Autodesk Inventor part; units mm, degrees
ref_plane "YZ Plane" through (0, 0, 0) normal (1, 0, 0) x (0, 1, 0)
ref_plane "XZ Plane" through (0, 0, 0) normal (0, 1, 0) x (-1, 0, 0)
ref_plane "XY Plane" through (0, 0, 0) normal (0, 0, 1) x (1, 0, 0)
sketch "Sketch1" plane through (0, 0, 0) normal (0, 1, 0) x (-1, 0, 0)
  circle A0 centre (0, 0) radius 8
  dimension "d0" = 16
extrude "Extrusion1" add sketch "Sketch1" along normal blind 7.1
sketch "Sketch2" plane through (0, 7.1, 0) normal (0, 1, 0) x (1, 0, 0)
  circle A0 centre (0, 0) radius 6
  dimension "d3" = 12
extrude "Extrusion2" add sketch "Sketch2" along normal blind 7.4
sketch "Sketch3" plane through (0, 14.5, 0) normal (0, 1, 0) x (1, 0, 0)
  circle A0 centre (0, 0) radius 8
extrude "Extrusion3" add sketch "Sketch3" along normal blind 1.5
chamfer "Chamfer1" distance 0.5 angle 45 4 edges at (-8, 16, 0) (-8, 14.5, 0) (8, 7.1, 0) (8, 0, 0)
sketch "Sketch4" plane through (0, 16, 0) normal (0, 1, 0) x (1, 0, 0)
  circle A0 centre (0, 0) radius 2.5
  dimension "d11" = 5
extrude "Extrusion4" cut sketch "Sketch4" against normal blind 16
properties part number "2GT_wheel"
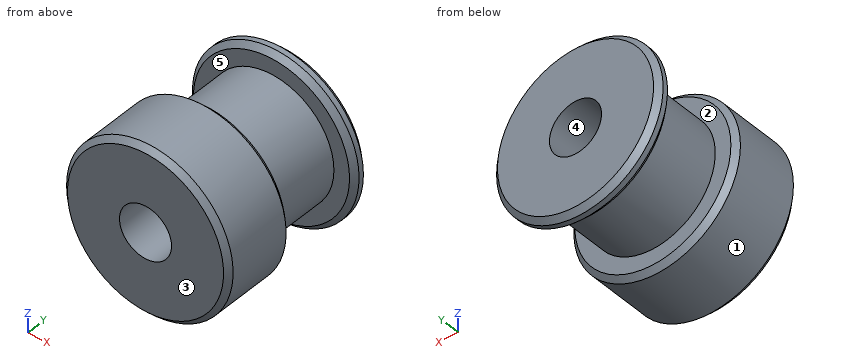
Design review of the part built by this model. Coordinates are the model's own, in mm. Face numbers are marked on the shaded views. A direction names the side the tool comes from. Round coordinates to 2 decimals unless told otherwise and drop trailing zeros. Loops run counter-clockwise (first coordinate to the right, second up) from the corner with the lowest first, then second, coordinate; pieces in that order, holes last. Notation, with made-up numbers: (68, 40) - (115, 40) arc R35 cw to (115, 74) - close; hole circle Ø4 at (26, 78.25). An arc over 180 degrees is marked (long way). One line per item, written item: value. Start each with the question number.
1) Consider section B-B on x = 0. Give the boundary of the cut face in (y, z), then the cut area to 3 significant figures.
2) Draft analysis for pull direction Y (two halves, no side actions). For the marked faces 3, 4 and 5, state which applies: +Y half, -Y half, draft (parallel to the pull), parting line (faces both ways), or undercut.
3) Consider section C-C on y = 7.5. Give the boundary of the cut face in (x, z).
4) For the marked faces 1 and 2, list the 3-axis set-ups (+Z, -Z, +X, -X, +Y, -Y) from which the entire face can be reached by the end or side of a thin tool; tool diameter is ignored.
5) To check wall thickness, follow L1, parallel to X at y = 12.25, z = 0; L2, parallel to Z at x = 0, y = 4.25. State the ranges of each line that lie inside material, in increasing order. Write a range as from..to.
6) Insertion check: pin 1 Ø2 at (y, z) = (3, -1.5) entering from -X; pin 2 Ø4 at (x, y) = (5, 11.5) entering from -Z; pin 3 Ø4 at (x, y) = (-4.5, 6.5) entering from -Z. Each pin has a flat end and moves straight along its axis. Give the tip position at first contact, or say it passes through.
7) Consider section A-A on z = 0. Give the boundary of the cut face in (x, y), then the cut area to 3 significant figures.
Reported:
1. outline: (0, -7.5) - (0.5, -8) - (6.6, -8) - (7.1, -7.5) - (7.1, -6) - (14.5, -6) - (14.5, -7.5) - (15, -8) - (15.5, -8) - (16, -7.5) - (16, -2.5) - (0, -2.5) - close; (0, 2.5) - (16, 2.5) - (16, 7.5) - (15.5, 8) - (15, 8) - (14.5, 7.5) - (14.5, 6) - (7.1, 6) - (7.1, 7.5) - (6.6, 8) - (0.5, 8) - (0, 7.5) - close
1. area: 145 mm^2
2. face 3: -Y half
2. face 4: draft
2. face 5: undercut
3. outline: circle Ø12 at (0, 0); hole circle Ø5 at (0, 0)
4. face 1: +Y, -Y
4. face 2: none
5. L1: x = -6..-2.5, 2.5..6
5. L2: z = -8..-2.5, 2.5..8
6. pin 1: stops at x = -7.98
6. pin 2: stops at z = -5.2
6. pin 3: stops at z = -7.6
7. outline: (-8, 0.5) - (-7.5, 0) - (-2.5, 0) - (-2.5, 16) - (-7.5, 16) - (-8, 15.5) - (-8, 15) - (-7.5, 14.5) - (-6, 14.5) - (-6, 7.1) - (-7.5, 7.1) - (-8, 6.6) - close; (2.5, 0) - (7.5, 0) - (8, 0.5) - (8, 6.6) - (7.5, 7.1) - (6, 7.1) - (6, 14.5) - (7.5, 14.5) - (8, 15) - (8, 15.5) - (7.5, 16) - (2.5, 16) - close
7. area: 145 mm^2
